Design review of the part built by this model. Coordinates are the model's own, in mm. Coordinates: 2 decimals unless noted, no trailing zeros. Loops run counter-clockwise (first coordinate to the right, second up) from the corner with the lowest first, then second, coordinate; pieces in that order, holes last. Notation, with made-up numbers: M -20,51.5 L 32,51.5 A10 ccw 32,69.5 Z; hole C 28,56.5 d5. An arc over 180 degrees is marked long. Write item = value, one per line. Start each with the question number.
Autodesk Fusion 360 part; units mm, degrees
sketch "Camber Block" plane through (0, 0, 0) normal (0, 0, 1) x (1, 0, 0)
  line L0 (0, 0) -> (2133.6, 0)
  line L1 (2133.6, 0) -> (2133.6, 101.6)
  line L2 (0, 0) -> (0, 101.6)
  arc A0 (2133.6, 101.6) -> (0, 101.6) centre (1066.8, -12352.7943) ccw
  circle A1 centre (50.8, 52.9209) radius 6.35
  circle A2 centre (152.4, 56.8518) radius 6.35
  circle A3 centre (254, 60.3684) radius 6.35
  circle A4 centre (355.6, 63.4708) radius 6.35
  line L3 (1066.8, 0) -> (1066.8, 147.2057) construction
  arc A5 (2133.6, 50.8) -> (0, 50.8) centre (1066.8, -24892.1929) ccw construction
  circle A6 centre (457.2, 66.1593) radius 6.35
  circle A7 centre (863.6, 72.7759) radius 6.35
  circle A8 centre (1270, 72.7759) radius 6.35
  circle A9 centre (1676.4, 66.1593) radius 6.35
  circle A10 centre (1778, 63.4708) radius 6.35
  circle A11 centre (1879.6, 60.3684) radius 6.35
  circle A12 centre (1981.2, 56.8518) radius 6.35
  circle A13 centre (2082.8, 52.9209) radius 6.35
  line L4 (416.8, 130.2942) -> (1716.8, 130.2942) construction
  dimension "BlockWidth" = 2133.6
  dimension "EndHeight" = 101.6
  dimension "CamberRadius" = 12500
  dimension "HoleDiameter" = 12.7
  dimension "d5" = 50.8
  dimension "d7" = 101.6
  dimension "d8" = 101.6
  dimension "d9" = 101.6
  dimension "d11" = 101.6
  dimension "d12" = 406.4
  dimension "TestLine" = 1300
  dimension "d16" = 22.5203
extrude "Extrude1" add sketch "Camber Block" along normal blind 19.05
equation "BlockWidth = 84\""
equation "EndHeight = 4\""
equation "d12 = 16\""

Autodesk Fusion 360 part; units mm, degrees
sketch "End Block Outline" plane through (0, 0, 0) normal (0, 0, 1) x (1, 0, 0)
  line L0 (0, 0) -> (0, 19.05)
  line L1 (0, 0) -> (279.4, 0) construction
  arc A0 (279.4, -3.123) -> (0, 0) centre (0, -12500) ccw
  arc A1 (0, 19.05) -> (195.4998, 97.9237) centre (0, 300.7741) ccw
  line L2 (0, 19.05) -> (279.4, 19.05) construction
  line L3 (279.4, 0) -> (279.4, -3.123) construction
  arc A2 (279.4, 62.2608) -> (195.4998, 97.9237) centre (229.8704, 62.2608) ccw
  line L4 (279.4, 62.2608) -> (279.4, -3.123)
  circle A3 centre (127, 22.225) radius 6.35
  circle A4 centre (228.6, 53.7591) radius 6.35
  line L5 (170, 19.05) -> (170, 76.1222) construction
  dimension "EndThickness" = 19.05
  dimension "BaseRadius" = 12500
  dimension "ArcRadius" = 281.7241
  dimension "BlockWidth" = 279.4
  dimension "ArcCordLength" = 210.8109
  dimension "d13" = 12.7
  dimension "d14" = 127
  dimension "d15" = 22.225
  dimension "d16" = 101.6
  dimension "d17" = 31.5341
  dimension "TestLength" = 170
  dimension "d2" = 65.002
extrude "Extrude1" add sketch "End Block Outline" along normal blind 19.05
equation "BlockWidth = 11\""
equation "ArcCordLength = 2 * ArcRadius * sin(ArcAngle / 2)"
equation "d14 = 5\""
equation "d15 = ( 7 / 8 ) * 1\""
equation "d16 = 4\""
equation "ArcLength = 216.06764 mm"
equation "ArcAngle = ( 360 * ArcLength / ( 2 * PI * ArcRadius ) ) * 1 deg"
(1) Take a section at B-B (x = 226). State the section outline as (y, z) points, plus the area to 3 significant figures.
(2) Insertion check: pin 1 (16.5 mm diameter, centred on x = 355.6, y = 63.47, fed in from -Z); pin 2 (2.5 mm diameter, centred on y = -2, z = 13.5, fed in from +X). Each pin has a flat end and moves straight along its axis. Give the tip position at first contact, or say it passes through.
(3) Take a section at C-C (x = 1037.5). State the section outline as (y, z) points, plus the area to 3 significant figures.
(4) To check wall thickness, follow L1, parallel to X at y = 75, z = 3; L2, parallel to X at y = 70, z = 16.25; L3, parallel to Y at x = 1981.2, z = 11.75. State the ranges of each line that lie inside material, in increasing order.
(5) Take a section at A-A (z = 7). Give the number of separate pieces and of enclosed holes in the cut face, plus the area to 3 significant figures.
Results list:
q1.outline = M -2.04,0 L 118.9,0 L 118.9,19.05 L -2.04,19.05 Z
q1.area = 2,300 mm^2
q2.pin_1 = 0
q2.pin_2 = 279.4
q3.outline = M 0,0 L 147.17,0 L 147.17,19.05 L 0,19.05 Z
q3.area = 2,800 mm^2
q4.L1 = 0 to 857.65, 869.55 to 1264.05, 1275.95 to 2133.6
q4.L2 = 0 to 452.14, 462.26 to 857.89, 869.31 to 1264.29, 1275.71 to 1671.34, 1681.46 to 2133.6
q4.L3 = 0 to 50.5, 63.2 to 113.72
q5.separate_pieces = 1
q5.enclosed_holes = 11
q5.area = 281,000 mm^2
